```python
from build123d import *

# Parameters (mm, degrees)
F0_W            = 396.24
F0_H            = 248.92
F1_DEPTH        = 21.59
F3_DEPTH        = 50.8
F5_DEPTH        = 63.5
F6_R            = 6.35
F7_R            = 5.08
F8_W            = 81.28
F8_H            = 137.16
F9_DEPTH        = 72.391
F10_W           = 50.8
F10_H           = 160.02
F11_DEPTH       = 10.414
F12_R           = 6.35
F13_R           = 19.05
F14_DEPTH       = 12.7
F15_SIZE        = 5.08
F17_D           = 7.1374
F17_DEPTH       = 127
F17_CSINK_D     = 13.4874
F17_CSINK_ANGLE = 82
F17_TIP         = 2.1442912911
F18_R           = 5.08
F20_D           = 12.7
F20_CBORE_D     = 22.225
F20_CBORE_DEPTH = 12.7
F21_R           = 19.05
F22_DEPTH       = 72.391
F24_SIZE        = 2.54
F25_R           = 25.4
F26_D           = 8.7376
F26_DEPTH       = 12.7
F26_TIP         = 2.6250398724


with BuildPart() as f1:
    # F0 (on Top) → F1 (new body)
    with BuildSketch(Plane.XY):
        Rectangle(F0_W, F0_H)
    extrude(amount=-F1_DEPTH)

    # F2 (on face) → F3 (join)
    with BuildSketch(Plane(origin=(0, 0, -21.59), x_dir=(1, 0, 0), z_dir=(0, 0, -1))):
        Polygon((127, 99.06), (-134.62, 99.06), (-134.62, -97.79), (95.25, -97.79), (95.25, -35.56), (127, -35.56), align=None)
    extrude(amount=F3_DEPTH)

    # F4 (on face) → F5 (cut)
    with BuildSketch(Plane.XY):
        Polygon((-116.84, -81.28), (109.22, -81.28), (109.22, 17.78), (77.47, 17.78), (77.47, 80.01), (-116.84, 80.01), align=None)
    extrude(amount=-F5_DEPTH, mode=Mode.SUBTRACT)

    # F6
    f6_edges = [f1.edges().sort_by_distance(p)[0] for p in [
        (-3.81, -81.28, -63.5),
        (109.22, -31.75, -63.5),
        (93.345, 17.78, -63.5),
        (77.47, 48.895, -63.5),
        (-19.685, 80.01, -63.5),
        (-116.84, -0.635, -63.5),
        (109.22, -81.28, -31.75),
        (-116.84, -81.28, -31.75),
        (-116.84, 80.01, -31.75),
        (109.22, 17.78, -31.75),
        (77.47, 80.01, -31.75),
    ]]
    fillet(f6_edges, radius=F6_R)

    # F7
    f7_edges = [f1.edges().sort_by_distance(p)[0] for p in [
        (95.25, 35.56, -46.99),
    ]]
    fillet(f7_edges, radius=F7_R)

    # F8 (on face) → F9 (cut, through all)
    with BuildSketch(Plane(origin=(0, 0, -72.39), x_dir=(1, 0, 0), z_dir=(0, 0, -1))):
        with Locations((-55.88, 0)):
            Rectangle(F8_W, F8_H)
    extrude(amount=-F9_DEPTH, mode=Mode.SUBTRACT)

    # F10 (on face) → F11 (cut)
    with BuildSketch(Plane.XY):
        with Locations((-161.29, 0)):
            Rectangle(F10_W, F10_H)
    extrude(amount=-F11_DEPTH, mode=Mode.SUBTRACT)

    # F12
    f12_edges = [f1.edges().sort_by_distance(p)[0] for p in [
        (-135.89, 0, -10.414),
        (-161.29, 80.01, -10.414),
        (-186.69, 0, -10.414),
        (-161.29, -80.01, -10.414),
        (-186.69, 80.01, -5.207),
        (-135.89, 80.01, -5.207),
        (-135.89, -80.01, -5.207),
        (-186.69, -80.01, -5.207),
    ]]
    fillet(f12_edges, radius=F12_R)

    # F13 (on face) → F14 (join)
    with BuildSketch(Plane.XY):
        with Locations((147.32, -73.66)):
            Circle(F13_R)
    extrude(amount=F14_DEPTH)

    # F15
    f15_edges = [f1.edges().sort_by_distance(p)[0] for p in [
        (128.27, -73.66, 12.7),
    ]]
    chamfer(f15_edges, length=F15_SIZE)

    # F17
    with Locations(Plane.XZ.offset(124.46)):
        with Locations((5.08, -10.668)):
            CounterSinkHole(F17_D / 2, F17_CSINK_D / 2, depth=F17_DEPTH, counter_sink_angle=F17_CSINK_ANGLE)
            with Locations((0, 0, -(F17_DEPTH + F17_TIP / 2))):  # 118° drill point
                Cone(0, F17_D / 2, F17_TIP, mode=Mode.SUBTRACT)

    # F18
    f18_edges = [f1.edges().sort_by_distance(p)[0] for p in [
        (-3.81, -99.06, -72.39),
        (-134.62, -99.06, -46.99),
        (-134.62, -0.635, -72.39),
        (127, -31.75, -72.39),
        (127, -99.06, -46.99),
        (127, 35.56, -46.99),
        (113.665, 35.56, -72.39),
        (95.25, 97.79, -46.99),
        (-19.685, 97.79, -72.39),
        (-134.62, 97.79, -46.99),
    ]]
    fillet(f18_edges, radius=F18_R)

    # F20 (through all)
    with Locations(Plane(origin=(0, 0, -21.59), x_dir=(1, 0, 0), z_dir=(0, 0, -1))):
        with Locations((-179.07, 105.41), (179.07, 105.41), (179.07, -105.41), (-179.07, -105.41)):
            CounterBoreHole(F20_D / 2, F20_CBORE_D / 2, F20_CBORE_DEPTH)

    # F21 (on face) → F22 (cut, through all)
    with BuildSketch(Plane.XY):
        with Locations((147.32, 73.66)):
            Circle(F21_R)
    extrude(amount=-F22_DEPTH, mode=Mode.SUBTRACT)

    # F24
    f24_edges = [f1.edges().sort_by_distance(p)[0] for p in [
        (198.12, 124.46, -10.795),
        (-198.12, 124.46, -10.795),
        (0, 124.46, 0),
        (0, 124.46, -21.59),
        (198.12, -124.46, -10.795),
        (198.12, 0, 0),
        (198.12, 0, -21.59),
        (-198.12, -124.46, -10.795),
        (-198.12, 0, 0),
        (-198.12, 0, -21.59),
        (90.17, 17.78, 0),
        (0, -124.46, -21.59),
        (0, -124.46, 0),
    ]]
    chamfer(f24_edges, length=F24_SIZE)

    # F25
    f25_edges = [f1.edges().sort_by_distance(p)[0] for p in [
        (-15.24, -68.58, -67.945),
        (-15.24, 68.58, -67.945),
        (-96.52, 68.58, -67.945),
        (-96.52, -68.58, -67.945),
    ]]
    fillet(f25_edges, radius=F25_R)

    # F26
    with Locations(Plane(origin=(-198.12, 0, 0), x_dir=(0, -1, 0), z_dir=(-1, 0, 0))):
        with Locations((-48.26, -11.7549253628), (27.94, -11.7549253628), (73.66, -11.7549253628), (-99.06, -11.7549253628)):
            Hole(F26_D / 2, depth=F26_DEPTH)
            with Locations((0, 0, -(F26_DEPTH + F26_TIP / 2))):  # 118° drill point
                Cone(0, F26_D / 2, F26_TIP, mode=Mode.SUBTRACT)


solid = f1.part
```
The model under review builds one solid part; all positions refer to its coordinate system, in mm. A direction names the side the tool comes from. Give positions to 0.01 mm unless a question says otherwise; leave off trailing zeros. Write each loop counter-clockwise with the first axis right and the second up, starting at its lowest first coordinate (ties: lowest second). Pieces come first, ordered by that corner, then holes. Notation, with made-up numbers: (-14.75, -28) -> (36.25, -28) arc R4 cw to (36.25, -21) -> close; hole circle Ø1 at (2.5, 50). An arc over 180 degrees is marked (long way). Answer in a Markdown table with one row per item.
1) Add section A-A on x = 179.07. State the section outline as (y, z) points.
Worked answers:
| item | result |
|---|---|
| outline | (-124.46, -19.05) -> (-121.92, -21.59) -> (-116.52, -21.59) -> (-116.52, -8.89) -> (-111.76, -8.89) -> (-111.76, 0) -> (-121.92, 0) -> (-124.46, -2.54) -> close; (-99.06, -8.89) -> (-94.3, -8.89) -> (-94.3, -21.59) -> (94.3, -21.59) -> (94.3, -8.89) -> (99.06, -8.89) -> (99.06, 0) -> (-99.06, 0) -> close; (111.76, -8.89) -> (116.52, -8.89) -> (116.52, -21.59) -> (121.92, -21.59) -> (124.46, -19.05) -> (124.46, -2.54) -> (121.92, 0) -> (111.76, 0) -> close |
2) Clearance check with flat-ended pins moving along their axes: P1, Ø6.5, axis at x = 176, y = 100, coming from the -Z side; P2, Ø19, axis at x = -159.5, y = 12, coming from the +Z side; P3, Ø7, axis at x = -62, z = -67.5, coming from the -Y side. State where each tip first meets the part, or that it passes through.
Worked answers:
| item | result |
|---|---|
| P1 | z = -8.89 |
| P2 | z = -10.41 |
| P3 | y = -99.06 |
3) Mouldability with a two-part tool opening along Y and no side actions: class faces 6 (the cylindrical face through (164.9, -81, 3.8)), 7 (the cylindrical face through (170.25, 112.17, -15.33)), 8 (the flat face through (127, -31, -44)), 9 (the flat face through (-15.24, 1, -68)) as +Y half, -Y half, draft (parallel to the pull), parting line (faces both ways), or undercut.
Worked answers:
| item | result |
|---|---|
| face 6 | parting line |
| face 7 | undercut |
| face 8 | draft |
| face 9 | undercut |
4) For L1, parallel to X at y = -104, z = -18; L2, parallel to Y at x = -179.07, z = -12.5; L3, parallel to Y at x = -9, z = -3, list the stretches that pass through material, from the lowest coordinate up. Write a range as [from, to].
Worked answers:
| item | result |
|---|---|
| L1 | [-198.12, -190.09], [-168.05, 168.05], [190.09, 198.12] |
| L2 | [-124.46, -116.52], [-94.3, 94.3], [116.52, 124.46] |
| L3 | [-124.46, -81.28], [80.01, 124.46] |
5) Add section C-C on x = -91.5. State the section outline as (y, z) points.
Worked answers:
| item | result |
|---|---|
| outline | (-124.46, -19.05) -> (-121.92, -21.59) -> (-99.06, -21.59) -> (-99.06, -67.31) arc R5.08 ccw to (-93.98, -72.39) -> (-58.34, -72.39) -> (-58.34, -63.5) -> (-74.93, -63.5) arc R6.35 cw to (-81.28, -57.15) -> (-81.28, -2.54) -> (-83.82, 0) -> (-121.92, 0) -> (-124.46, -2.54) -> close; (58.34, -72.39) -> (92.71, -72.39) arc R5.08 ccw to (97.79, -67.31) -> (97.79, -21.59) -> (121.92, -21.59) -> (124.46, -19.05) -> (124.46, -2.54) -> (121.92, 0) -> (82.55, 0) -> (80.01, -2.54) -> (80.01, -57.15) arc R6.35 cw to (73.66, -63.5) -> (58.34, -63.5) -> close |
6) Add section D-D on x = 46.5. State the section outline as (y, z) points, plus the area to 3 significant figures.
Worked answers:
| item | result |
|---|---|
| outline | (-124.46, -19.05) -> (-121.92, -21.59) -> (-99.06, -21.59) -> (-99.06, -67.31) arc R5.08 ccw to (-93.98, -72.39) -> (92.71, -72.39) arc R5.08 ccw to (97.79, -67.31) -> (97.79, -21.59) -> (121.92, -21.59) -> (124.46, -19.05) -> (124.46, -2.54) -> (121.92, 0) -> (82.55, 0) -> (80.01, -2.54) -> (80.01, -57.15) arc R6.35 cw to (73.66, -63.5) -> (-74.93, -63.5) arc R6.35 cw to (-81.28, -57.15) -> (-81.28, -2.54) -> (-83.82, 0) -> (-121.92, 0) -> (-124.46, -2.54) -> close |
| area | 5,120 mm² |
7) Tool access review of faces 1 (the flat face through (-3, 124.46, -11)), 2 (the flat face through (-5, -81.28, -29)), 3 (the flat face through (-21, 97.79, -44)), 4 (the flat face through (-174, 110, -8.89)), 5 (the cylindrical face through (-22.88, 61.34, -67.88)): name each direction out of +Z, -Z, +X, -X, +Y, -Y from which nothing blocks a thin tool from reaching the whole face with its end or side.
Worked answers:
| item | result |
|---|---|
| face 1 | +Z, -Z, +X, -X, +Y |
| face 2 | +Z |
| face 3 | -Z, +X, -X, +Y |
| face 4 | -Z |
| face 5 | +Z, -Z |
